Geometry: final body of the model. Coordinates: model frame, mm. Coordinates: 2 decimals unless noted, no trailing zeros. Order: outer loops, then holes, each group sorted by start corner. A loop starts at its lowest first (then second) coordinate and runs counter-clockwise, first axis right, second up. Notation, with made-up numbers: M 25,-11 L 61,-11 A13 ccw 61,6 Z; hole C 84,27 d5. An arc over 180 degrees is marked long. Use CSV: the item, a comma, the result in double quotes. Start each with the question number.
1. Pull-direction query (Y, two-part tool) for faces 1 (the flat face through (0, 0, 0)), 2 (the cylindrical face through (1.9, 6.8, -1)), 3 (the cylindrical face through (0.08, 9.67, -0.99)); classes: pulls with the +Y half, pulls with the -Y half, needs draft (parallel to the pull), parting line crosses it, or undercut.
2. Section query C-C on z = -1.45. Return the cut outline in (x, y), and give its area (3 significant figures).
3. Section query A-A on x = 0. Return the cut outline in (y, z).
4. Section query B-B on y = 7.25. Return the cut outline in (x, z).
5. Material intervals for line 1 (Y direction, x = 0, z = -0.55); line 2 (Y direction, x = -1.25, z = -0.6); line 3 (X direction, y = 8, z = -1.1), sorted ascending.
6. Section query D-D on x = -2.5. Return the cut outline in (y, z), and give its area (3 significant figures).
Autodesk Inventor part; units mm, degrees
ref_plane "YZ Plane" through (0, 0, 0) normal (1, 0, 0) x (0, 1, 0)
ref_plane "XZ Plane" through (0, 0, 0) normal (0, 1, 0) x (-1, 0, 0)
ref_plane "XY Plane" through (0, 0, 0) normal (0, 0, 1) x (1, 0, 0)
sketch "Skizze1" plane through (0, 0, 0) normal (0, 0, 1) x (1, 0, 0)
  line L0 (3.5, 6.171) -> (3.5, -6.171)
  line L1 (3.5, -6.171) -> (-3.5, -6.171)
  line L2 (-3.5, -6.171) -> (-3.5, 6.171)
  arc A0 (3.5, 6.171) -> (-3.5, 6.171) centre (0, 6.171) ccw
  circle A1 centre (0, 6.171) radius 2
  point P0 (0, 0)
  point P1 (-3.5, 0)
extrude "Extrusion1" add sketch "Skizze1" against normal blind 2
properties part number "planetenstab"
Results list:
1,face 1,"needs draft"
1,face 2,"undercut"
1,face 3,"pulls with the +Y half"
2,outline,"M -3.5,-6.17 L 3.5,-6.17 L 3.5,6.17 A3.5 ccw -3.5,6.17 Z; hole C 0,6.17 d4"
2,area,"93.1 mm²"
3,outline,"M -6.17,-2 L 4.17,-2 L 4.17,0 L -6.17,0 Z; M 8.17,-2 L 9.67,-2 L 9.67,0 L 8.17,0 Z"
4,outline,"M -3.33,-2 L -1.68,-2 L -1.68,0 L -3.33,0 Z; M 1.68,-2 L 3.33,-2 L 3.33,0 L 1.68,0 Z"
5,line 1,"y = -6.17 to 4.17, 8.17 to 9.67"
5,line 2,"y = -6.17 to 4.61, 7.73 to 9.44"
5,line 3,"x = -2.98 to -0.81, 0.81 to 2.98"
6,outline,"M -6.17,-2 L 8.62,-2 L 8.62,0 L -6.17,0 Z"
6,area,"29.6 mm²"
